Autodesk Fusion 360 part; units mm, degrees
sketch "Skizze1" plane through (0, 0, 0) normal (0, 0, 1) x (1, 0, 0)
  circle A0 centre (0, 0) radius 17
  dimension "d1" = 34
extrude "Extrusion1" add sketch "Skizze1" along normal blind 9.5
sketch "Skizze2" plane through (0, 0, 9.5) normal (0, 0, 1) x (-1, 0, 0)
  circle A0 centre (0, 0) radius 17
  circle A1 centre (0, 0) radius 20
  dimension "d5" = 40
extrude "Extrusion2" add sketch "Skizze2" along normal blind 3 contours A0 | A1
sketch "Skizze3" plane through (0, 0, 0) normal (0, 0, -1) x (1, 0, 0)
  circle A0 centre (0, 0) radius 17
  circle A1 centre (0, 0) radius 20
  dimension "d8" = 40
extrude "Extrusion3" add sketch "Skizze3" along normal blind 3 contours A0 | A1
Can you work these out from the model? Positions are in its coordinate system, mm. A direction names the side the tool comes from. Give positions to 0.01 mm unless a question says otherwise; leave off trailing zeros. Loops run counter-clockwise (first coordinate to the right, second up) from the corner with the lowest first, then second, coordinate; pieces in that order, holes last. Notation, with made-up numbers: (81.25, 71.5) - (118.25, 71.5) arc R20 ccw to (118.25, 96.5) - close; hole circle Ø10 at (30, 57.5). An arc over 180 degrees is marked (long way). One line per item, written item: value.
(1) If we section it at D-D, the plane z = 8.25: List the corners of the cut face in (x, y) for me, plus the area to 3 significant figures.
Verdict:
outline: circle Ø34 at (0, 0)
area: 908 mm^2
(2) I need wall thicknesses on line 1 along Z through (x, y) = (-15.5, 10); line 2 along Y through (x, z) = (0, 4); line 3 along X through (y, z) = (2.5, -0.25). Which ranges of each line are inside material? Lowest first, please.
Verdict:
line 1: -3 to 0, 9.5 to 12.5
line 2: -17 to 17
line 3: -19.84 to 19.84
(3) If we section it at C-C, the plane z = -1.5: List the corners of the cut face in (x, y) for me.
Verdict:
outline: circle Ø40 at (0, 0)
(4) On a 3-axis mill with a long thin cutter (end or side, diameter ignored), from which of +Z, -Z, +X, -X, +Y, -Y can I reach the whole of each face in a straight line? I mean faces 5 (the face through (4.336, -19.524, 10.979)), 6 (the face through (9.139, -14.334, 4.684)). Say none if no direction works.
Verdict:
face 5: +Z, -Z
face 6: none
(5) I'm going to push flat-ended pins straight in: pin 1 (8 mm diameter, centred on y = 3.5, z = 3, fed in from -X); pin 2 (4 mm diameter, centred on y = -6, z = 1.5, fed in from +X); pin 3 (3 mm diameter, centred on y = 15.5, z = 0.5, fed in from -X). Where does each tip first touch, or does it pass through?
Verdict:
pin 1: x = -19.98
pin 2: x = 19.45
pin 3: x = -14.2
(6) If we mould it in two halves opening along Z, with no side actions, what happens to faces 1 (the face through (0, 0, -3)), 2 (the face through (0, 0, 12.5)), 3 (the face through (-9, 15, 0)), 4 (the face through (-4.336, -19.524, -1.479))? For each: released by +Z, released by -Z, zero draft, split by the parting line, or undercut.
Verdict:
face 1: released by -Z
face 2: released by +Z
face 3: undercut
face 4: zero draft
(7) If we section it at A-A, the plane y = 0: List the corners of the cut face in (x, z) for me.
Verdict:
outline: (-20, -3) - (20, -3) - (20, 0) - (17, 0) - (17, 9.5) - (20, 9.5) - (20, 12.5) - (-20, 12.5) - (-20, 9.5) - (-17, 9.5) - (-17, 0) - (-20, 0) - close
